Work out the finished part from the listing and answer in its coordinate system (mm). A direction names the side the tool comes from. Round coordinates to 2 decimals unless told otherwise and drop trailing zeros. Write each loop counter-clockwise with the first axis right and the second up, starting at its lowest first coordinate (ties: lowest second). Pieces come first, ordered by that corner, then holes. Notation, with made-up numbers: (58.25, -26.5) - (64.25, -26.5) arc R18 cw to (64.25, -9.5) - close; hole circle Ø8 at (19.5, 71.5). An arc over 180 degrees is marked (long way). Answer as a JSON object with one key per item and string values.
```python
from build123d import *

# Parameters (mm, degrees)
BOSS_EXTRUDE2_DEPTH = 35.7124
CUT_EXTRUDE1_REACH  = 66.642
SKETCH3_R           = 4.1656
CUT_EXTRUDE2_REACH  = 66.642
SKETCH5_R           = 4.1656
SKETCH6_R           = 9.525
CUT_EXTRUDE3_DEPTH  = 47.498
SKETCH7_R           = 9.525
CUT_EXTRUDE4_DEPTH  = 47.498


with BuildPart() as part:
    # Sketch2 → Boss-Extrude2 (new, symmetric)
    with BuildSketch(Plane.XY):
        with BuildLine():
            Line((0, 38.1), (0, 0))
            Line((0, 0), (38.1, 0))
            Line((38.1, 0), (38.1, 3.719743879))
            ThreePointArc((38.1, 3.719743879), (37.616635031, 6.149783674), (36.240128061, 8.209871939))
            Line((36.240128061, 8.209871939), (8.209871939, 36.240128061))
            ThreePointArc((8.209871939, 36.240128061), (6.149783674, 37.616635031), (3.719743879, 38.1))
            Line((3.719743879, 38.1), (0, 38.1))
        make_face()
        with BuildLine():
            Line((6.35, 27.893323389), (6.35, 6.858))
            ThreePointArc((6.35, 6.858), (6.498789755, 6.498789755), (6.858, 6.35))
            Line((6.858, 6.35), (27.893323389, 6.35))
            ThreePointArc((27.893323389, 6.35), (28.362654192, 6.663596816), (28.252533634, 7.217210245))
            Line((28.252533634, 7.217210245), (7.217210245, 28.252533634))
            ThreePointArc((7.217210245, 28.252533634), (6.663596816, 28.362654192), (6.35, 27.893323389))
        make_face(mode=Mode.SUBTRACT)
    extrude(amount=BOSS_EXTRUDE2_DEPTH, both=True)

    # Sketch3 → Cut-Extrude1 (cut, up to next)
    with BuildSketch(Plane.ZY, mode=Mode.PRIVATE) as cut_extrude1_sk1:
        with Locations(Location((19.05, 19.05, 0), (0, 0, 270))):
            Circle(SKETCH3_R)
    cut_extrude1_tool1 = extrude(cut_extrude1_sk1.sketch, amount=-CUT_EXTRUDE1_REACH, mode=Mode.PRIVATE) & part.part
    # Sketch3 → Cut-Extrude1 (cut, up to next)
    with BuildSketch(Plane.ZY, mode=Mode.PRIVATE) as cut_extrude1_sk2:
        with Locations(Location((-19.05, 19.05, 0), (0, 0, 90))):
            Circle(SKETCH3_R)
    cut_extrude1_tool2 = extrude(cut_extrude1_sk2.sketch, amount=-CUT_EXTRUDE1_REACH, mode=Mode.PRIVATE) & part.part
    add(cut_extrude1_tool1.solids().sort_by_distance((0, 19.05, 19.05))[0], mode=Mode.SUBTRACT)
    add(cut_extrude1_tool2.solids().sort_by_distance((0, 19.05, -19.05))[0], mode=Mode.SUBTRACT)

    # Sketch5 → Cut-Extrude2 (cut, up to next)
    with BuildSketch(Plane.XZ, mode=Mode.PRIVATE) as cut_extrude2_sk1:
        with Locations(Location((19.05, 19.05, 0), (0, 0, 270))):
            Circle(SKETCH5_R)
    cut_extrude2_tool1 = extrude(cut_extrude2_sk1.sketch, amount=-CUT_EXTRUDE2_REACH, mode=Mode.PRIVATE) & part.part
    # Sketch5 → Cut-Extrude2 (cut, up to next)
    with BuildSketch(Plane.XZ, mode=Mode.PRIVATE) as cut_extrude2_sk2:
        with Locations(Location((19.05, -19.05, 0), (0, 0, 180))):
            Circle(SKETCH5_R)
    cut_extrude2_tool2 = extrude(cut_extrude2_sk2.sketch, amount=-CUT_EXTRUDE2_REACH, mode=Mode.PRIVATE) & part.part
    add(cut_extrude2_tool1.solids().sort_by_distance((19.05, 0, 19.05))[0], mode=Mode.SUBTRACT)
    add(cut_extrude2_tool2.solids().sort_by_distance((19.05, 0, -19.05))[0], mode=Mode.SUBTRACT)

    # Sketch6 → Cut-Extrude3 (cut)
    with BuildSketch(Plane(origin=(6.35, 0, 0), x_dir=(0, 0, -1), z_dir=(1, 0, 0))):
        with Locations(Location((-19.05, 19.05, 0), (0, 0, 111.808163998))):
            Circle(SKETCH6_R)
        with Locations(Location((19.05, 19.05, 0), (0, 0, 111.808163998))):
            Circle(SKETCH6_R)
    extrude(amount=CUT_EXTRUDE3_DEPTH, mode=Mode.SUBTRACT)

    # Sketch7 → Cut-Extrude4 (cut)
    with BuildSketch(Plane(origin=(0, 6.35, 0), x_dir=(1, 0, 0), z_dir=(0, 1, 0))):
        with Locations((19.05, 19.05)):
            Circle(SKETCH7_R)
        with Locations((19.05, -19.05)):
            Circle(SKETCH7_R)
    extrude(amount=CUT_EXTRUDE4_DEPTH, mode=Mode.SUBTRACT)


solid = part.part
```
Item 1: A cutting plane is placed at D-D (x = 20.5). Give the number of separate pieces and of enclosed holes in the cut face, and give its area (3 significant figures).
Results found:
{"separate pieces": "6", "enclosed holes": "0", "area": "657 mm²"}
Item 2: A cutting plane is placed at A-A (z = 30). Write down the section's boundary in (x, y), and give its area (3 significant figures).
Results found:
{"outline": "(0, 0) - (38.1, 0) - (38.1, 3.72) arc R6.35 ccw to (36.24, 8.21) - (8.21, 36.24) arc R6.35 ccw to (3.72, 38.1) - (0, 38.1) - close; hole (6.35, 6.86) arc R0.51 ccw to (6.86, 6.35) - (27.89, 6.35) arc R0.51 ccw to (28.25, 7.22) - (7.22, 28.25) arc R0.51 ccw to (6.35, 27.89) - close", "area": "687 mm²"}
Item 3: Consider line 1 along Z through (x, y) = (25, 19.05) (3 decimals); line 2 along Z through (x, y) = (22, 4.5); line 3 along X through (y, z) = (27.25, 19.05). Determine where each line is inside the solid, lowest interval first.
Results found:
{"line 1": "-35.712 to -28.575, -9.525 to 9.525, 28.575 to 35.712", "line 2": "-35.71 to -21.99, -16.11 to 16.11, 21.99 to 35.71", "line 3": "0 to 6.35"}
Item 4: For faces 4 (the cylindrical face through (28.707, 9.633, 20.478)), 5 (the flat face through (17.88, 17.59, 0.23)), 6 (the cylindrical face through (28.508, 9.378, 17.923)), determine the directions among +Z, -Z, +X, -X, +Y, -Y from which every point of the face is accessible in a straight line to the end or side of a thin tool.
Results found:
{"face 4": "+X", "face 5": "+Z, -Z", "face 6": "+Y"}
Item 5: A cutting plane is placed at C-C (z = 19.05). Write down the section's boundary in (x, y) (3 decimals), and give its area (3 significant figures).
Results found:
{"outline": "(0, 0) - (14.884, 0) - (14.884, 6.35) - (6.858, 6.35) arc R0.508 cw to (6.35, 6.858) - (6.35, 14.884) - (0, 14.884) - close; (0, 23.216) - (6.35, 23.216) - (6.35, 28.575) - (9.525, 28.575) - (9.525, 34.925) - (8.21, 36.24) arc R6.35 ccw to (3.72, 38.1) - (0, 38.1) - close; (23.216, 0) - (38.1, 0) - (38.1, 3.72) arc R6.35 ccw to (36.24, 8.21) - (34.925, 9.525) - (28.575, 9.525) - (28.575, 6.35) - (23.216, 6.35) - close", "area": "386 mm²"}
Item 6: A cutting plane is placed at B-B (x = 14). Write down the section's boundary in (y, z) (3 decimals), and give its area (3 significant figures).
Results found:
{"outline": "(0, -35.712) - (6.35, -35.712) - (6.35, 35.712) - (0, 35.712) - close; (21.47, -35.712) - (30.45, -35.712) - (30.45, -27.126) - (24.1, -27.126) arc R9.525 cw to (21.47, -28.263) - close; (21.47, -9.837) arc R9.525 cw to (24.1, -10.974) - (30.45, -10.974) - (30.45, 10.974) - (24.1, 10.974) arc R9.525 cw to (21.47, 9.837) - close; (21.47, 28.263) arc R9.525 cw to (24.1, 27.126) - (30.45, 27.126) - (30.45, 35.712) - (21.47, 35.712) - close", "area": "798 mm²"}
Item 7: Each of these flat-tipped pins is pushed along its axis until it touches: P1, Ø6.5, axis at x = 19.05, z = 19.05, coming from the +Y side; P2, Ø2, axis at x = 12.5, z = 15.5, coming from the +Y side; P3, Ø22, axis at y = 19.05, z = 19.05, coming from the +X side; P4, Ø17, axis at y = 19.05, z = 19.05, coming from the +X side. Where does it stop, or does it pass through?
Results found:
{"P1": "through", "P2": "y = 6.35", "P3": "x = 36.39", "P4": "x = 6.35"}
Item 8: Determine the mould class of faces 1 (the cylindrical face through (3.13, 22.36, 16.52)), 2 (the flat face through (19, 19, -35.712)), 3 (the flat face through (2, 38.1, 0)) for opening direction Y: pulls with the +Y half, pulls with the -Y half, needs draft (parallel to the pull), parting line crosses it, or undercut.
Results found:
{"face 1": "undercut", "face 2": "needs draft", "face 3": "pulls with the +Y half"}
